```python
from build123d import *

# Parameters (mm, degrees)
CROQUIS1_W              = 101.9
CROQUIS1_H              = 126
SALIENTE_EXTRUIR1_DEPTH = 15
VACIADO1_T              = -3
CORTAR_EXTRUIR1_DEPTH   = 15
CROQUIS3_W              = 8
CROQUIS3_H              = 39
CORTAR_EXTRUIR2_DEPTH   = 15
CROQUIS4_W              = 47.2
CROQUIS4_H              = 7
CORTAR_EXTRUIR3_DEPTH   = 15
CROQUIS5_R              = 1.4
CORTAR_EXTRUIR4_DEPTH   = 15
SALIENTE_EXTRUIR2_START = 12
CROQUIS6_R              = 4.4
CROQUIS6_R_2            = 1.4
SALIENTE_EXTRUIR2_DEPTH = 12
CROQUIS7_W              = 101.9
CROQUIS7_H              = 126
CROQUIS7_W_2            = 95.9
CROQUIS7_H_2            = 120
SALIENTE_EXTRUIR3_DEPTH = 5


with BuildPart() as part:
    # Croquis1 → Saliente-Extruir1 (new body)
    with BuildSketch(Plane.XY):
        with Locations((50.95, 63)):
            Rectangle(CROQUIS1_W, CROQUIS1_H)
    extrude(amount=SALIENTE_EXTRUIR1_DEPTH)

    # Vaciado1
    vaciado1_openings = [part.faces().sort_by_distance(p)[0] for p in [
        (50.95, 63, 15),
    ]]
    offset(amount=VACIADO1_T, openings=vaciado1_openings, kind=Kind.INTERSECTION)

    # Croquis2 → Cortar-Extruir1 (cut)
    with BuildSketch(Plane.XY.offset(3)):
        Polygon((5.1, 37.3), (81.1, 37.3), (81.1, 23.3), (97.1, 23.3), (97.1, 5.3), (5.1, 5.3), align=None)
    extrude(amount=-CORTAR_EXTRUIR1_DEPTH, mode=Mode.SUBTRACT)

    # Croquis3 → Cortar-Extruir2 (cut)
    with BuildSketch(Plane(origin=(101.9, 0, 0), x_dir=(0, 0, -1), z_dir=(1, 0, 0))):
        with Locations((-7.5, 59.5)):
            Rectangle(CROQUIS3_W, CROQUIS3_H)
    extrude(amount=-CORTAR_EXTRUIR2_DEPTH, mode=Mode.SUBTRACT)

    # Croquis4 → Cortar-Extruir3 (cut)
    with BuildSketch(Plane(origin=(0, 126, 0), x_dir=(1, 0, 0), z_dir=(0, 1, 0))):
        with Locations((37.6, -7.5)):
            Rectangle(CROQUIS4_W, CROQUIS4_H)
    extrude(amount=-CORTAR_EXTRUIR3_DEPTH, mode=Mode.SUBTRACT)

    # Croquis5 → Cortar-Extruir4 (cut)
    with BuildSketch(Plane.XY.offset(3)):
        with Locations((8.07, 117.93)):
            Circle(CROQUIS5_R)
        with Locations((93.83, 117.93)):
            Circle(CROQUIS5_R)
    extrude(amount=-CORTAR_EXTRUIR4_DEPTH, mode=Mode.SUBTRACT)

    # Croquis6 → Saliente-Extruir2 (add)
    # profile 1 of 2: a face of its own
    with BuildSketch(Plane.XY.offset(3).offset(SALIENTE_EXTRUIR2_START)):
        with Locations(Location((93.83, 117.93, 0), (0, 0, 180))):
            Circle(CROQUIS6_R)
        with Locations((93.83, 117.93)):
            Circle(CROQUIS6_R_2, mode=Mode.SUBTRACT)
    # profile 2 of 2: a face of its own
    with BuildSketch(Plane.XY.offset(3).offset(SALIENTE_EXTRUIR2_START)):
        with Locations(Location((8.07, 117.93, 0), (0, 0, 180))):
            Circle(CROQUIS6_R)
        with Locations((8.07, 117.93)):
            Circle(CROQUIS6_R_2, mode=Mode.SUBTRACT)
    extrude(amount=-SALIENTE_EXTRUIR2_DEPTH)

    # Croquis7 → Saliente-Extruir3 (add)
    with BuildSketch(Plane.XY.offset(15)):
        with Locations((50.95, 63)):
            Rectangle(CROQUIS7_W, CROQUIS7_H)
        with Locations((50.95, 63)):
            Rectangle(CROQUIS7_W_2, CROQUIS7_H_2, mode=Mode.SUBTRACT)
    extrude(amount=SALIENTE_EXTRUIR3_DEPTH)


solid = part.part
```
Source: CAD feature listing. Evaluate the final solid. Frame: model axes, mm. A direction names the side the tool comes from. Round coordinates to 2 decimals unless told otherwise and drop trailing zeros. Write each loop counter-clockwise with the first axis right and the second up, starting at its lowest first coordinate (ties: lowest second). Pieces come first, ordered by that corner, then holes. Notation, with made-up numbers: M -30,28 L 21,28 A16 cw 21,36 Z; hole C 46,33 d3. An arc over 180 degrees is marked long. Answer as a JSON object with one key per item and string values. Group by question number.
(1) Ray query, line 1 (Y direction, x = 93.83, z = 8); line 2 (X direction, y = 117.93, z = 6); line 3 (X direction, y = 5, z = 17.5). Return the intervals inside material, ascending. Write a range as [from, to].
(2) Reachability of faces 1 (the flat face through (3, 62, 11)), 2 (the flat face through (97.1, 14, 2)), 3 (the flat face through (37, 125, 4)), 4 (the flat face through (100, 79, 8)), 5 (the flat face through (2, 63, 20)) from +Z, -Z, +X, -X, +Y, -Y: full face, straight path, thin tool, end or side. Return the list, or none.
(3) Section query B-B on y = 32.5. Output: boundary loops of the cut face in (x, z).
(4) Section query D-D on y = 117.93. Output: boundary loops of the cut face in (x, z), then the cut area to 3 significant figures.
(5) Section query A-A on z = 7.75. Output: boundary loops of the cut face in (x, y), then the cut area to 3 significant figures.
(6) First-contact query: pin 1 (1.5 mm diameter, centred on x = 100.5, z = 6, fed in from -Y); pin 2 (10 mm diameter, centred on x = 38, y = 102, fed in from +Z); pin 3 (3 mm diameter, centred on x = 93.83, y = 117.93, fed in from +Z). Flat tips, straight axial feed; report the tip coordinate or a pass-through.
(7) Mould query, pull axis Y, two halves, no side actions, for faces 6 (the flat face through (61.2, 125, 8)), 7 (the flat face through (100, 40, 8)), 8 (the flat face through (50, 126, 12)). Classes: +Y half, -Y half, draft (parallel to the pull), parting line (faces both ways), or undercut.
(8) Section query C-C on x = 93.83. Output: boundary loops of the cut face in (y, z), then the cut area to 3 significant figures.
Computed values:
{
 "1": {"line 1": "[0, 3], [113.53, 116.53], [119.33, 122.33], [123, 126]", "line 2": "[0, 3], [3.67, 6.67], [9.47, 12.47], [89.43, 92.43], [95.23, 98.23], [98.9, 101.9]", "line 3": "[0, 3], [98.9, 101.9]"},
 "2": {"face 1": "+Z", "face 2": "+Z, -Z", "face 3": "+Y", "face 4": "+X", "face 5": "+Z, +X, -X, +Y, -Y"},
 "3": {"outline": "M 0,0 L 5.1,0 L 5.1,3 L 3,3 L 3,20 L 0,20 Z; M 81.1,0 L 101.9,0 L 101.9,20 L 98.9,20 L 98.9,3 L 81.1,3 Z"},
 "4": {"outline": "M 0,0 L 6.67,0 L 6.67,15 L 3.67,15 L 3.67,3 L 3,3 L 3,20 L 0,20 Z; M 9.47,0 L 92.43,0 L 92.43,15 L 89.43,15 L 89.43,3 L 12.47,3 L 12.47,15 L 9.47,15 Z; M 95.23,0 L 101.9,0 L 101.9,20 L 98.9,20 L 98.9,3 L 98.23,3 L 98.23,15 L 95.23,15 Z", "area": "535 mm^2"},
 "5": {"outline": "M 0,0 L 101.9,0 L 101.9,40 L 98.9,40 L 98.9,3 L 3,3 L 3,123 L 14,123 L 14,126 L 0,126 Z; C 8.07,117.93 d8.8; M 61.2,123 L 98.9,123 L 98.9,79 L 101.9,79 L 101.9,126 L 61.2,126 Z; C 93.83,117.93 d8.8; hole C 8.07,117.93 d2.8; hole C 93.83,117.93 d2.8", "area": "1,180 mm^2"},
 "6": {"pin 1": "y = 0", "pin 2": "z = 3", "pin 3": "z = 15"},
 "7": {"face 6": "draft", "face 7": "undercut", "face 8": "+Y half"},
 "8": {"outline": "M 0,0 L 5.3,0 L 5.3,3 L 3,3 L 3,20 L 0,20 Z; M 23.3,0 L 116.53,0 L 116.53,15 L 113.53,15 L 113.53,3 L 23.3,3 Z; M 119.33,0 L 126,0 L 126,20 L 123,20 L 123,3 L 122.33,3 L 122.33,15 L 119.33,15 Z", "area": "490 mm^2"}
}
